The model under review builds one solid part; all positions refer to its coordinate system, in mm. A direction names the side the tool comes from. Round coordinates to 2 decimals unless told otherwise and drop trailing zeros. Write each loop counter-clockwise with the first axis right and the second up, starting at its lowest first coordinate (ties: lowest second). Pieces come first, ordered by that corner, then holes. Notation, with made-up numbers: (39.5, -7.5) - (66.5, -7.5) arc R3 ccw to (66.5, -3.5) - close; hole circle Ø11 at (-27.75, 23). An arc over 180 degrees is marked (long way). Use one line per item in the form item = value.
from build123d import *

# Parameters (mm, degrees)
F0_W          = 31.6
F0_H          = 17.6
F1_DEPTH      = 25
F2_W          = 30
F2_H          = 16
F3_DEPTH      = 23.5
F4_R          = 22
F5_DEPTH      = 12.6
F5_DEPTH_BACK = 15.801
F6_W          = 25
F6_H          = 50
F7_DEPTH      = 3.2


with BuildPart() as f1:
    # F0 (on Top) → F1 (new body)
    with BuildSketch(Plane.XY):
        Rectangle(F0_W, F0_H)
    extrude(amount=F1_DEPTH)

    # F2 (on face) → F3 (cut)
    with BuildSketch(Plane.XY.offset(25)):
        Rectangle(F2_W, F2_H)
    extrude(amount=-F3_DEPTH, mode=Mode.SUBTRACT)

    # F4 (on Right) → F5 (cut, two sides)
    with BuildSketch(Plane.YZ) as f5_sk:
        with Locations((0, 31.5)):
            Circle(F4_R)
    extrude(amount=F5_DEPTH, mode=Mode.SUBTRACT)
    extrude(f5_sk.sketch, amount=-F5_DEPTH_BACK, mode=Mode.SUBTRACT)

    # F6 (on face) → F7 (cut)
    with BuildSketch(Plane.YZ.offset(15.8)):
        with Locations((0, 34.5)):
            Rectangle(F6_W, F6_H)
    extrude(amount=-F7_DEPTH, mode=Mode.SUBTRACT)


solid = f1.part
(1) To check wall thickness, follow L1, parallel to X at y = -6, z = 2; L2, parallel to Y at x = 11.5, z = 6.5; L3, parallel to Z at x = 5.5, y = 3.25. State the ranges of each line that lie inside material, in increasing order.
Geometry results:
L1 = -15.8 to -15, 15 to 15.8
L2 = -8.8 to -8, 8 to 8.8
L3 = 0 to 1.5
(2) Insertion check: P1, Ø2.5, axis at x = 13.5, y = -2.5, coming from the +Z side; P2, Ø0.9, axis at y = -8.5, z = 10.5, coming from the +X side. Each pin has a flat end and moves straight along its axis. Give the tip position at first contact, or say it passes through.
Geometry results:
P1 = 1.5
P2 = 12.6
(3) The part is to be moulded in two halves that separate along Y. For faces 1 (the flat face through (0, 8.8, 6)), 2 (the flat face through (-15, 0, 6)), 3 (the flat face through (15.8, 0, 5)), 4 (the flat face through (0, -8, 6)), say which applies: +Y half, -Y half, draft (parallel to the pull), parting line (faces both ways), or undercut.
Geometry results:
face_1 = +Y half
face_2 = undercut
face_3 = draft
face_4 = undercut
(4) Add section C-C on x = -10. Write out the cut boundary in (y, z).
Geometry results:
outline = (-8.8, 0) - (8.8, 0) - (8.8, 11.34) arc R22 cw to (8, 11.01) - (8, 1.5) - (-8, 1.5) - (-8, 11.01) arc R22 cw to (-8.8, 11.34) - close
(5) Add section B-B on y = 0. Write out the cut boundary in (x, z).
Geometry results:
outline = (-15.8, 0) - (15.8, 0) - (15.8, 9.5) - (15, 9.5) - (15, 1.5) - (-15, 1.5) - (-15, 9.5) - (-15.8, 9.5) - close
(6) Add section A-A on z = 6.75. Write out the cut boundary in (x, y).
Geometry results:
outline = (-15.8, -8.8) - (15.8, -8.8) - (15.8, 8.8) - (-15.8, 8.8) - close; hole (-15, -8) - (15, -8) - (15, 8) - (-15, 8) - close
(7) Machinability: for faces 5 (the flat face through (0, 8, 6)), 6 (the flat face through (-15.8, 0, 6)), 7 (the flat face through (12.6, -8.4, 10.4)), which of the approach directions +Z, -Z, +X, -X, +Y, -Y give a long, thin tool a straight path to every point of the face, cutting with its end or side? Answer none if there is none.
Geometry results:
face_5 = +Z
face_6 = +Z, -Z, -X, +Y, -Y
face_7 = +Z, +X, +Y, -Y
